Can you work these out from the drawing? Everything is in mm from the part's minimum corner. A direction names the side the tool comes from. Round coordinates to 2 decimals unless told otherwise and drop trailing zeros. Write each loop counter-clockwise with the first axis right and the second up, starting at its lowest first coordinate (ties: lowest second). Pieces come first, ordered by that corner, then holes. Notation, with made-up numbers: (73, 39) -> (109, 39) arc R12 cw to (109, 47) -> close; hole circle Ø6 at (-7.5, 62.25). An arc over 180 degrees is marked (long way). One line per question, with ' | ' between items. Start each with the question number.
1. Imagine slicing it at A-A, the plane z = 19. List the corners of the cut face in (x, y) for me, and give its area (3 significant figures).
2. For the marked faces 5 and 6, which set-ups out of +Z, -Z, +X, -X, +Y, -Y let a thin tool reach every point of the face, with its end or its side?
3. Imagine slicing it at D-D, the plane y = 13. State how many separate pieces and enclosed holes the cut face has, and give its area (3 significant figures).
4. Thinking about a two-plate mould opening in X: for the marked faces 1, 2, 3 and 4, which applies, released by +X, released by -X, zero draft, split by the parting line, or undercut?
5. If I drill on line 1 along X through (y, z) = (20, 19); line 2 along X through (y, z) = (34, 19); line 3 along Z through (x, y) = (120.4, 17.75), over which ranges is the centre line in solid material (lowest first)? Write a range as [from, to].
6. Imagine slicing it at C-C, the plane x = 120.4. List the corners of the cut face in (y, z) for me, and give its area (3 significant figures).
7. For pin 1 Ø6 at (x, y) = (40, 23) entering from +Z; pin 2 Ø5 at (x, z) = (120.4, 19) entering from +Y; pin 3 Ø6 at (x, z) = (75, 29) entering from -Y, each with a flat end and sliding along its axis, tell me the tip position at first contact or that it passes through.
8. Imagine slicing it at B-B, the plane y = 19. List the corners of the cut face in (x, z) for me, and give its area (3 significant figures).
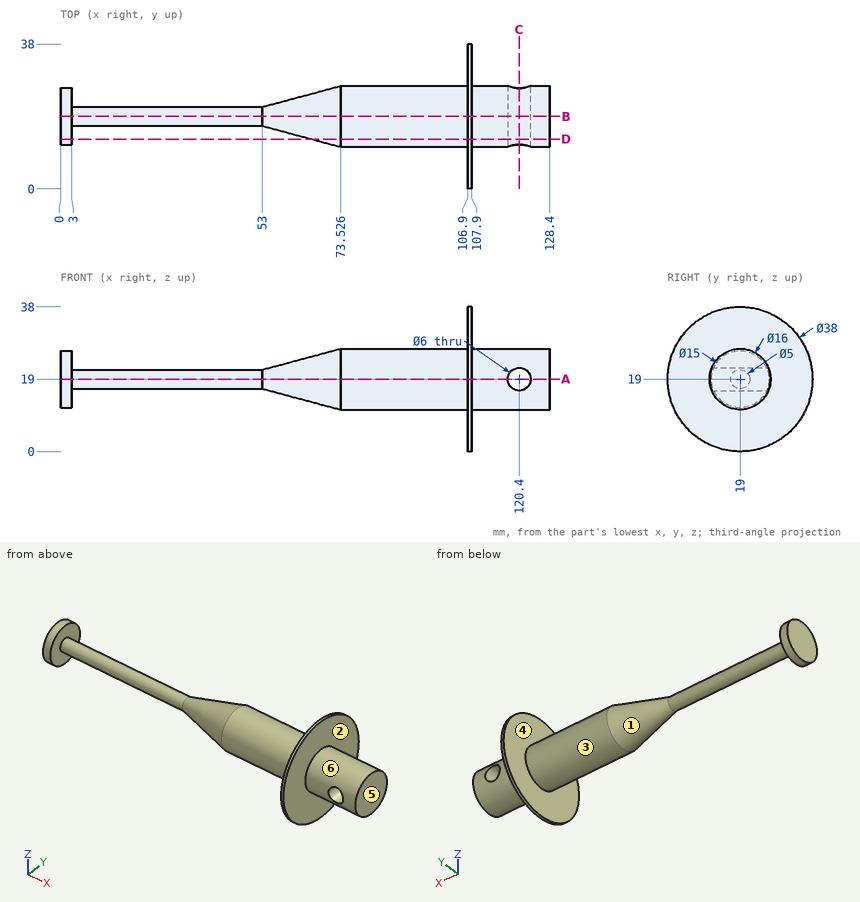
Geometry results:
1) outline: (0, 11.5) -> (3, 11.5) -> (3, 16.5) -> (53, 16.5) -> (73.53, 11) -> (106.9, 11) -> (106.9, 0) -> (107.9, 0) -> (107.9, 11) -> (117.4, 11) -> (117.4, 27) -> (107.9, 27) -> (107.9, 38) -> (106.9, 38) -> (106.9, 27) -> (73.53, 27) -> (53, 21.5) -> (3, 21.5) -> (3, 26.5) -> (0, 26.5) -> close; (123.4, 11) -> (128.4, 11) -> (128.4, 27) -> (123.4, 27) -> close | area: 1,310 mm2
2) face 5: +Z, -Z, +X, +Y, -Y | face 6: +X
3) separate pieces: 2 | enclosed holes: 1 | area: 656 mm2
4) face 1: undercut | face 2: released by +X | face 3: zero draft | face 4: released by -X
5) line 1: x = [0, 117.4], [123.4, 128.4] | line 2: x = [106.9, 107.9] | line 3: z = [11.1, 16], [22, 26.9]
6) outline: (11.58, 16) arc R8 ccw to (26.42, 16) -> close; (11.58, 22) -> (26.42, 22) arc R8 ccw to start | area: 107 mm2
7) pin 1: stops at z = 21.29 | pin 2: passes through | pin 3: stops at y = 15.13
8) outline: (0, 11.5) -> (3, 11.5) -> (3, 16.5) -> (53, 16.5) -> (73.53, 11) -> (106.9, 11) -> (106.9, 0) -> (107.9, 0) -> (107.9, 11) -> (128.4, 11) -> (128.4, 27) -> (107.9, 27) -> (107.9, 38) -> (106.9, 38) -> (106.9, 27) -> (73.53, 27) -> (53, 21.5) -> (3, 21.5) -> (3, 26.5) -> (0, 26.5) -> close; hole circle Ø6 at (120.4, 19) | area: 1,380 mm2
